Print and shaded views of the part. All mm, measured from the part's lowest x, y and z. Coordinates: 2 decimals unless noted, no trailing zeros. Loops run counter-clockwise (first coordinate to the right, second up) from the corner with the lowest first, then second, coordinate; pieces in that order, holes last. Notation, with made-up numbers: M -10,78.5 L 39,78.5 A22 ccw 39,87.5 Z; hole C 28,-19 d7. An arc over 180 degrees is marked long. Answer as CSV lines item,"result". Start each with the question number.
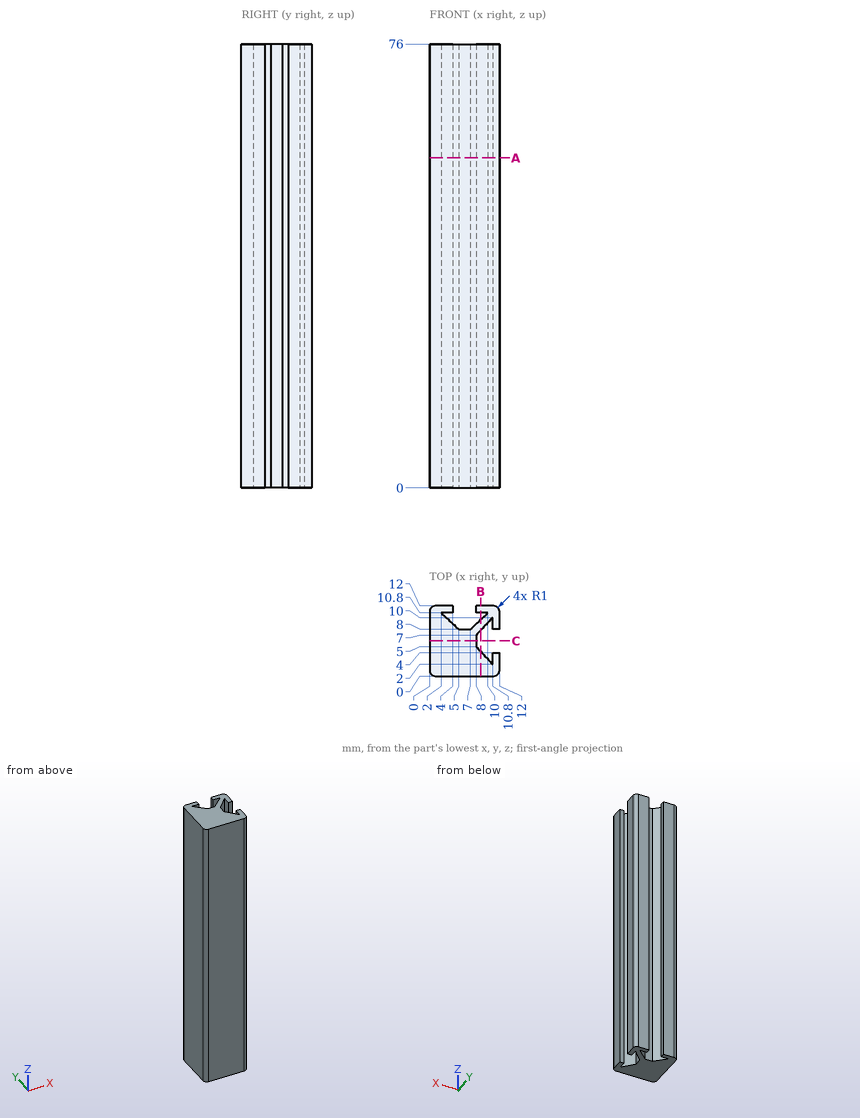
Q1. Wall check: L1, parallel to X at y = 9, z = 23.5; L2, parallel to X at y = 5.5, z = 45.5; L3, parallel to Y at x = 8.75, z = 49.5. Give the ranges that are in metal, low to high.
Q2. Slice it at C-C, the plane y = 6. Write the cut outline in (x, z).
Q3. Slice it at A-A, the plane z = 56.5. Write the cut outline in (x, y).
Q4. Slice it at B-B, the plane x = 8.75. Write the cut outline in (y, z), and give its area (3 significant figures).
Q5. Flat gauge pins, fed straight in: P1, Ø0.6, axis at y = 6, z = 51.5, coming from the +X side; P2, Ø1.6, axis at x = 6, z = 34.5, coming from the +Y side; P3, Ø0.6, axis at y = 11.5, z = 51.5, coming from the +X side. Where does each tip first touch, or does it go through?
Solved:
1,L1,"x = 0 to 3.93, 8.07 to 9.87, 10.8 to 12"
1,L2,"x = 0 to 8"
1,L3,"y = 0 to 4.2, 7.8 to 9.63, 10.8 to 12"
2,outline,"M 0,0 L 8,0 L 8,76 L 0,76 Z"
3,outline,"M 0,1 A1 ccw 1,0 L 11,0 A1 ccw 12,1 L 12,4 L 10.8,4 L 10.8,2 L 8,5 L 8,7 L 10.8,10 L 10.8,8 L 12,8 L 12,11 A1 ccw 11,12 L 8,12 L 8,10.8 L 10,10.8 L 7,8 L 5,8 L 2,10.8 L 4,10.8 L 4,12 L 1,12 A1 ccw 0,11 Z"
4,outline,"M 0,0 L 4.2,0 L 4.2,76 L 0,76 Z; M 7.8,0 L 9.63,0 L 9.63,76 L 7.8,76 Z; M 10.8,0 L 12,0 L 12,76 L 10.8,76 Z"
4,area,"549 mm2"
5,P1,"stops at x = 8"
5,P2,"stops at y = 8"
5,P3,"stops at x = 11.98"
